Input: dimensioned drawing with shaded views. Units: mm. Origin: part minimum x, y, z. A direction names the side the tool comes from. Round coordinates to 2 decimals unless told otherwise and drop trailing zeros. Write each loop counter-clockwise with the first axis right and the second up, starting at its lowest first coordinate (ties: lowest second). Pieces come first, ordered by that corner, then holes. Notation, with made-up numbers: (-33.5, 66) - (-10.5, 66) arc R29 cw to (-10.5, 95) - close; hole circle Ø5 at (33, 12). An arc over 180 degrees is marked (long way). Use one line per item in the form item = value.
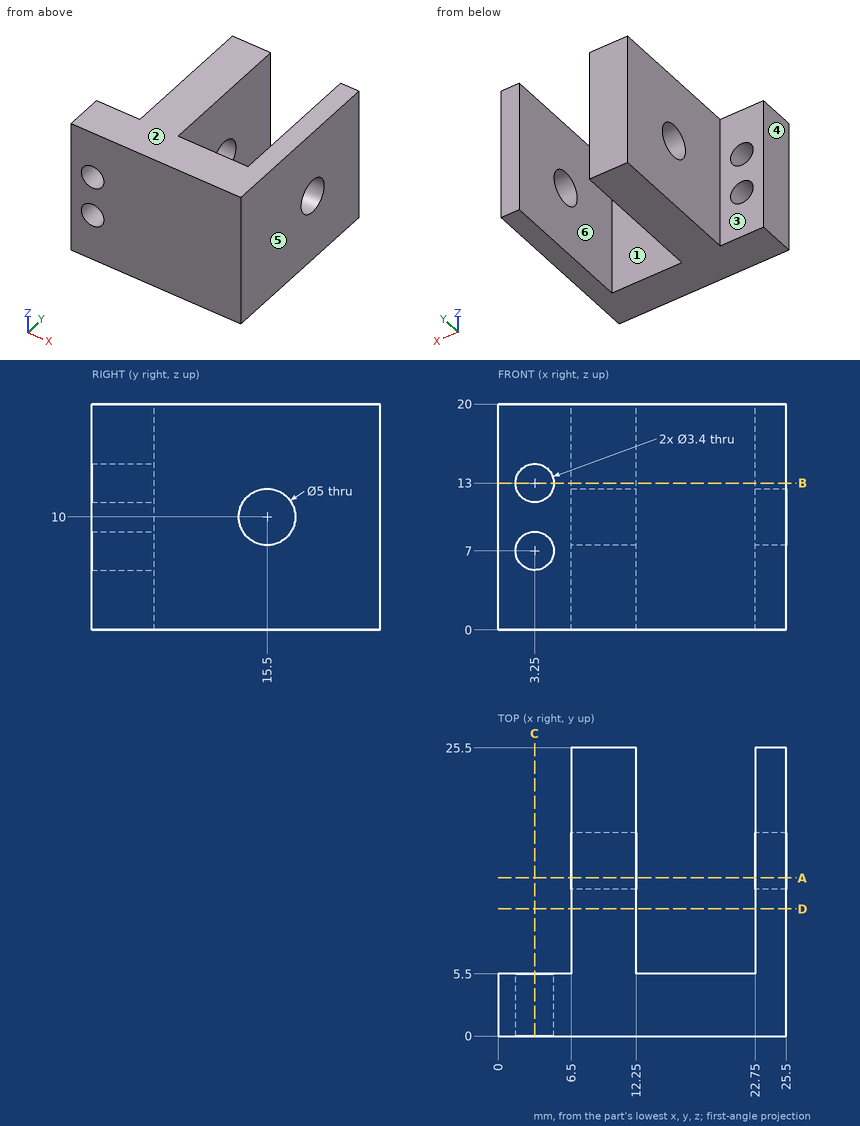
(1) First-contact query: pin 1 Ø2.5 at (x, z) = (3.25, 7) entering from +Y; pin 2 Ø3 at (y, z) = (21, 17.5) entering from -X; pin 3 Ø5 at (x, z) = (3, 5) entering from +Y. Flat tips, straight axial feed; report the tip coordinate or a pass-through.
Derived:
pin_1 = through
pin_2 = 6.5
pin_3 = 5.5
(2) Material intervals for L1, parallel to Z at x = 3.25, y = 4.1; L2, parallel to X at y = 24, z = 10; L3, parallel to Y at x = 24.5, z = 10, sorted ascending.
Derived:
L1 = 0 to 5.3, 8.7 to 11.3, 14.7 to 20
L2 = 6.5 to 12.25, 22.75 to 25.5
L3 = 0 to 13, 18 to 25.5
(3) Cut plane C-C on x = 3.25. Output: boundary loops of the cut face in (y, z).
Derived:
outline = (0, 0) - (5.5, 0) - (5.5, 5.3) - (0, 5.3) - close; (0, 8.7) - (5.5, 8.7) - (5.5, 11.3) - (0, 11.3) - close; (0, 14.7) - (5.5, 14.7) - (5.5, 20) - (0, 20) - close
(4) Cut plane B-B on z = 13. Output: boundary loops of the cut face in (x, y), then the cut area to 3 significant figures.
Derived:
outline = (0, 0) - (1.55, 0) - (1.55, 5.5) - (0, 5.5) - close; (4.95, 0) - (25.5, 0) - (25.5, 25.5) - (22.75, 25.5) - (22.75, 5.5) - (12.25, 5.5) - (12.25, 25.5) - (6.5, 25.5) - (6.5, 5.5) - (4.95, 5.5) - close
area = 292 mm^2
(5) Access query for the marked faces 1, 2 and 3. Directions: +Z, -Z, +X, -X, +Y, -Y. A direction counts if a zero-diameter tool reaches every point of the face in a straight line with its end or side. Return the directions, or none.
Derived:
face_1 = +Z, -Z, +Y
face_2 = +Z, +X, -X, +Y, -Y
face_3 = +Z, -Z, -X, +Y
(6) Cut plane A-A on y = 14. Output: boundary loops of the cut face in (x, z).
Derived:
outline = (6.5, 0) - (12.25, 0) - (12.25, 8) - (6.5, 8) - close; (6.5, 12) - (12.25, 12) - (12.25, 20) - (6.5, 20) - close; (22.75, 0) - (25.5, 0) - (25.5, 8) - (22.75, 8) - close; (22.75, 12) - (25.5, 12) - (25.5, 20) - (22.75, 20) - close
(7) Draft query along X for the marked faces 4, 5 and 6. Return one class per face: released by +X, released by -X, zero draft, split by the parting line, or undercut.
Derived:
face_4 = released by -X
face_5 = released by +X
face_6 = undercut
(8) Cut plane D-D on y = 11.25. Output: boundary loops of the cut face in (x, z), then the cut area to 3 significant figures.
Derived:
outline = (6.5, 0) - (12.25, 0) - (12.25, 20) - (6.5, 20) - close; (22.75, 0) - (25.5, 0) - (25.5, 20) - (22.75, 20) - close
area = 170 mm^2
